from build123d import *

# Parameters (mm, degrees)
EXTRUDE1_DEPTH                              = 9.525
SKETCH5_R                                   = 3.175
EXTRUDE2_DEPTH                              = 251.181385449
CIRPATTERN1_COUNT                           = 6
TAPPED_HOLE_FOR_10_32_HELICOIL1_D           = 5.1054
TAPPED_HOLE_FOR_10_32_HELICOIL1_CBORE_D     = 5.93598
TAPPED_HOLE_FOR_10_32_HELICOIL1_CBORE_DEPTH = 8.556


with BuildPart() as part:
    # Sketch1 → Extrude1 (new body)
    with BuildSketch(Plane(origin=(0, 0, 0), x_dir=(1, 0, 0), z_dir=(0, 1, 0))):
        with BuildLine():
            Line((-175, -150), (175, -150))
            ThreePointArc((175, -150), (192.67766953, -142.67766953), (200, -125))
            Line((200, -125), (200, 125))
            ThreePointArc((200, 125), (192.67766953, 142.67766953), (175, 150))
            Line((175, 150), (-175, 150))
            ThreePointArc((-175, 150), (-192.67766953, 142.67766953), (-200, 125))
            Line((-200, 125), (-200, -125))
            ThreePointArc((-200, -125), (-192.67766953, -142.67766953), (-175, -150))
        make_face()
    extrude(amount=EXTRUDE1_DEPTH)

    # Sketch5 → Extrude2 (cut, through all)
    with BuildSketch(Plane(origin=(0, 9.525, 0), x_dir=(1, 0, 0), z_dir=(0, 1, 0))):
        with Locations(Location((-62.5, 22.525, 0), (0, 0, 270))):
            Circle(SKETCH5_R)
    extrude(amount=-EXTRUDE2_DEPTH, mode=Mode.SUBTRACT)

    # Sketch3 → CSK for 1/4 Flat Head Machine Screw1 (revolve, cut)
    with BuildSketch(Plane(origin=(-189.5, 9.525, -22.525), x_dir=(0, 0, 1), z_dir=(1, 0, 0))):
        Polygon((0, 0), (0, 9.525), (3.3782, 9.525), (3.3782, 4.520932584), (6.4389, 1), (6.4389, 0), align=None)
    csk_for_1_4_flat_head_machine_screw1 = revolve(axis=Axis((-189.5, 15.875, -22.525), (0, -1, 0)), mode=Mode.SUBTRACT)

    # CirPattern1: CSK for 1/4 Flat Head Machine Screw1 ×6 about axis
    cirpattern1_axis = Axis((-62.5, 0, -22.525), (0, 1, 0))
    for i in range(1, CIRPATTERN1_COUNT):
        add(csk_for_1_4_flat_head_machine_screw1.rotate(cirpattern1_axis, i * 360 / CIRPATTERN1_COUNT), mode=Mode.SUBTRACT)

    # Tapped Hole for #10-32 Helicoil1 (through all)
    with Locations(Plane(origin=(0, 9.525, 0), x_dir=(-1, 0, 0), z_dir=(0, 1, 0))):
        with Locations((-141, 85), (141, -85), (141, 0), (141, 85), (-141, -85), (-141, 0)):
            CounterBoreHole(TAPPED_HOLE_FOR_10_32_HELICOIL1_D / 2, TAPPED_HOLE_FOR_10_32_HELICOIL1_CBORE_D / 2, TAPPED_HOLE_FOR_10_32_HELICOIL1_CBORE_DEPTH)


solid = part.part
Input: part model. Units: mm. Frame: model coordinates. A direction names the side the tool comes from. Give positions to 0.01 mm unless a question says otherwise; leave off trailing zeros. Answer as a JSON object with one key per item and string values. Group by question number.
Item 1: Pin query (flat end, axial travel): P1, Ø7.5, axis at x = -141, z = 85, coming from the -Y side; P2, Ø11, axis at x = 1, z = -132.51, coming from the +Y side; P3, Ø7.5, axis at x = 1, z = -132.51, coming from the +Y side; P4, Ø5.5, axis at x = 141, z = 85, coming from the +Y side. Return the tip coordinate at first contact, or that it passes through.
Item 2: Line query: probe 1 along Z at (x, y) = (-126, 8.8); probe 2 along Z at (x, y) = (-3.5, 7.25); probe 3 along Z at (x, y) = (141, 0.3). Output: solid intervals per line, ascending.
Item 3: Reachability of faces 1 (the cylindrical face through (6.712, 9.032, -129.539)), 2 (the cylindrical face through (192.871, 4.696, -142.482)) from +Z, -Z, +X, -X, +Y, -Y: full face, straight path, thin tool, end or side. Return the list, or none.
Item 4: Pull-direction query (Z, two-part tool) for faces 3 (the cylindrical face through (0.717, 9.032, 81.028)), 4 (the flat face through (200, 5, 2)), 5 (the flat face through (2, 5, -150)); classes: released by +Z, released by -Z, zero draft, split by the parting line, or undercut.
Checks:
{
 "1": {"P1": "stops at y = 0", "P2": "stops at y = 7.45", "P3": "stops at y = 5.43", "P4": "stops at y = 0.97"},
 "2": {"probe 1": "z = -150 to -138.95, -126.07 to 81.02, 93.9 to 150", "probe 2": "z = -150 to -135.37, -129.65 to 84.6, 90.32 to 150", "probe 3": "z = -150 to -87.55, -82.45 to -2.55, 2.55 to 82.45, 87.55 to 150"},
 "3": {"face 1": "+Y", "face 2": "-Z, +X, +Y, -Y"},
 "4": {"face 3": "undercut", "face 4": "zero draft", "face 5": "released by -Z"}
}
